Check sheet for the drawn part. Datum: minimum x, y, z corner. Units: mm. A direction names the side the tool comes from. Give positions to 0.01 mm unless a question says otherwise; leave off trailing zeros. Write each loop counter-clockwise with the first axis right and the second up, starting at its lowest first coordinate (ties: lowest second). Pieces come first, ordered by that corner, then holes. Notation, with made-up numbers: (65, 10.25) - (84, 10.25) arc R11 ccw to (84, 27.25) - close; hole circle Ø10 at (29, 2.25). An arc over 180 degrees is marked (long way). Answer as a JSON object with one key per item and string values. Group by question number.
Item 1: Scan lines: line 1 along X through (y, z) = (1.25, 12.5); line 2 along Z through (x, y) = (24.5, 10); line 3 along Y through (x, z) = (13, 5.75). Record each from-to range of solid material in increasing order. Write a range as [from, to].
Item 2: Draft check along Z on the marked faces 1, 2, 3 and 4. Enter one of: +Z half, -Z half, draft (parallel to the pull), parting line (faces both ways), or undercut.
Item 3: Sectioned sample at C-C, the plane y = 4.5. Record the boundary of the cut face in (x, z).
Item 4: Tool access check on the marked faces 5, 6 and 7. Record the directions out of +Z, -Z, +X, -X, +Y, -Y that give a thin tool (end or side, any length) a straight path to the whole face; none if there is none.
Item 5: Go/stop test with flat-tipped pins: pin 1 (3 mm diameter, centred on x = 13.5, z = 12.5, fed in from +Y); pin 2 (3 mm diameter, centred on y = 18.5, z = 11.5, fed in from -X); pin 3 (15 mm diameter, centred on y = 24, z = 12, fed in from -X); pin 4 (1.8 mm diameter, centred on x = 15, z = 13, fed in from +Y). Record where each tip stops, or that it passes through.
Item 6: Sectioned sample at A-A, the plane y = 18.5. Record the boundary of the cut face in (x, z).
Item 7: Sectioned sample at B-B, the plane x = 13.5. Record the boundary of the cut face in (y, z), and give its area (3 significant figures).
Item 8: Sectioned sample at D-D, the plane x = 18. Record the boundary of the cut face in (y, z).
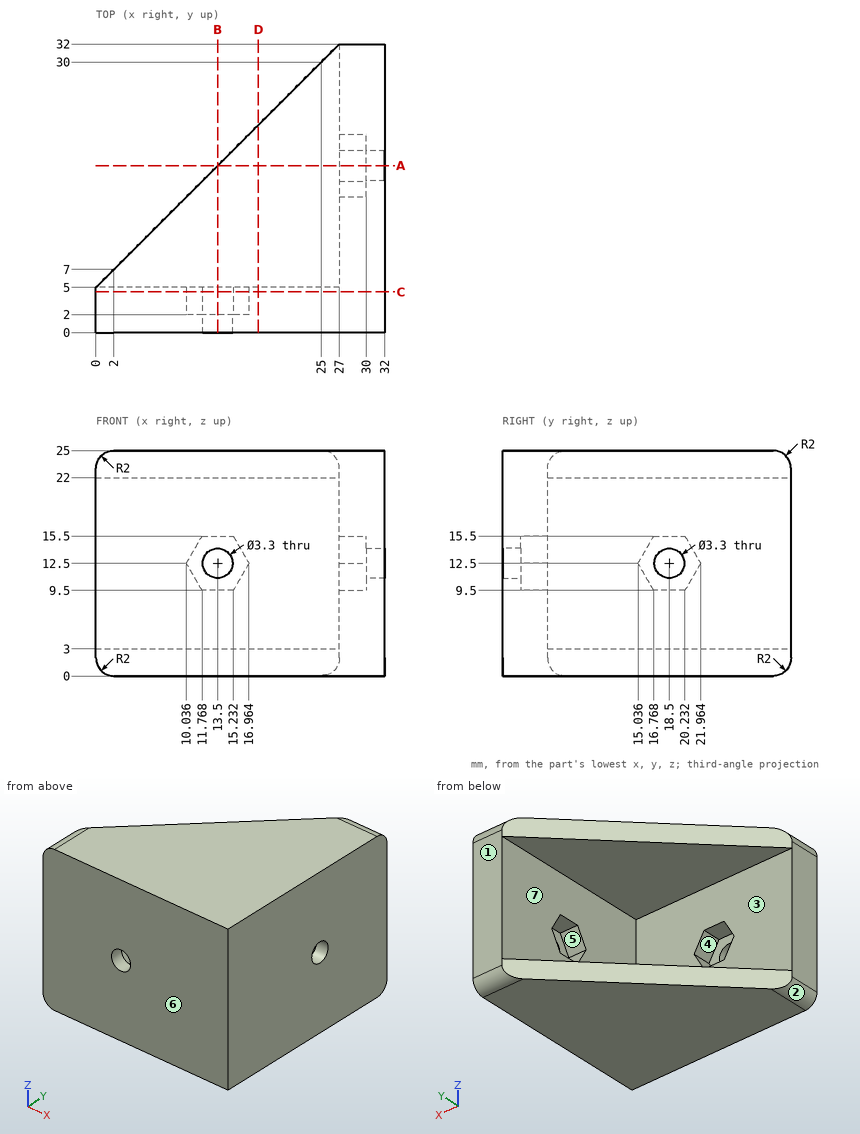
Geometry check:
{
 "1": {"line 1": "[0, 11.85], [15.15, 32]", "line 2": "[0, 3], [22, 25]", "line 3": "[0, 5]"},
 "2": {"face 1": "draft", "face 2": "-Z half", "face 3": "undercut", "face 4": "undercut"},
 "3": {"outline": "(0, 2) arc R2 ccw to (2, 0) - (32, 0) - (32, 25) - (2, 25) arc R2 ccw to (0, 23) - close; hole (10.04, 12.5) - (11.77, 9.5) - (15.23, 9.5) - (16.96, 12.5) - (15.23, 15.5) - (11.77, 15.5) - close"},
 "4": {"face 5": "-X", "face 6": "+Z, -Z, +X, -X, -Y", "face 7": "-X, +Y"},
 "5": {"pin 1": "through", "pin 2": "x = 30", "pin 3": "x = 27", "pin 4": "y = 2"},
 "6": {"outline": "(13.5, 0) - (32, 0) - (32, 10.85) - (30, 10.85) - (30, 9.5) - (27, 9.5) - (27, 3) - (13.5, 3) - close; (13.5, 22) - (27, 22) - (27, 15.5) - (30, 15.5) - (30, 14.15) - (32, 14.15) - (32, 25) - (13.5, 25) - close"},
 "7": {"outline": "(0, 0) - (18.5, 0) - (18.5, 3) - (5, 3) - (5, 9.5) - (2, 9.5) - (2, 10.85) - (0, 10.85) - close; (0, 14.15) - (2, 14.15) - (2, 15.5) - (5, 15.5) - (5, 22) - (18.5, 22) - (18.5, 25) - (0, 25) - close", "area": "181 mm^2"},
 "8": {"outline": "(0, 0) - (23, 0) - (23, 3) - (5, 3) - (5, 22) - (23, 22) - (23, 25) - (0, 25) - close"}
}
